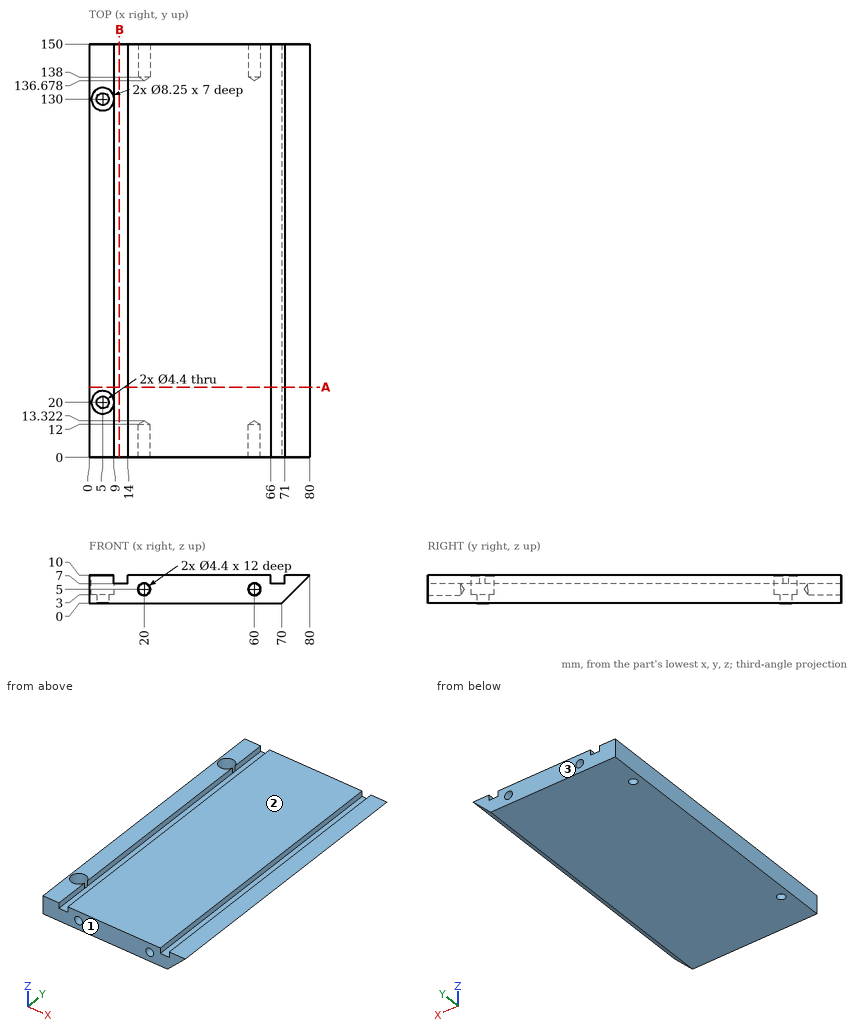
Drawing for the job (mm, zero at the part's lowest x, y, z). Round coordinates to 2 decimals unless told otherwise and drop trailing zeros. Order: outer loops, then holes, each group sorted by start corner. A loop starts at its lowest first (then second) coordinate and runs counter-clockwise, first axis right, second up.
Item 1: Probe line 1 along Y through (x, z) = (5, 6.75) (3 decimals); line 2 along Y through (x, z) = (5, 1.95); line 3 along Z through (x, y) = (60, 141). List the from-to ranges inside material, lowest first.
Item 2: Saw through at A-A on y = 25.5. Write the cut outline in (x, z).
Item 3: Pin check, flat tips, straight feed: pin 1 (5 mm diameter, centred on y = 114, z = 6, fed in from +X); pin 2 (3.5 mm diameter, centred on y = 9.5, z = 8, fed in from +X); pin 3 (2.5 mm diameter, centred on y = 105, z = 8, fed in from +X). Stop position of each tip, or through.
Item 4: Saw through at B-B on x = 11. Write the cut outline in (y, z).
Item 5: Mould opens along Y. For the marked faces 1, 2 and 3 say: pulls with the +Y half, pulls with the -Y half, needs draft (parallel to the pull), parting line crosses it, or undercut.
Reported:
1. line 1: y = 0 to 15.875, 24.125 to 125.875, 134.125 to 150
1. line 2: y = 0 to 17.8, 22.2 to 127.8, 132.2 to 150
1. line 3: z = 0 to 2.8, 7.2 to 10
2. outline: (0, 0) - (70, 0) - (80, 10) - (71, 10) - (71, 7) - (66, 7) - (66, 10) - (14, 10) - (14, 7) - (9, 7) - (9, 10) - (0, 10) - close
3. pin 1: stops at x = 78.5
3. pin 2: stops at x = 79.75
3. pin 3: stops at x = 79.25
4. outline: (0, 0) - (150, 0) - (150, 7) - (0, 7) - close
5. face 1: pulls with the -Y half
5. face 2: needs draft
5. face 3: pulls with the +Y half
